from build123d import *

# Parameters (mm, degrees)
SKETCH1_W                                = 70.104
SKETCH1_H                                = 38.1
RECTANGULAR_BASE_DEPTH                   = 3.175
SKETCH2_R                                = 34.29
CIRCULAR_BASE_ADD_ON_DEPTH               = 3.175
HOLE_FOR_SERVO_ARM_DEPTH                 = 4.175
TAB_DEPTH                                = 3.175
CIRCULAR_PATTERN_OF_SERVO_ARM_HOLE_COUNT = 4
SKETCH6_R                                = 11.43
CUT_EXTRUDE2_DEPTH                       = 4.175


with BuildPart() as part:
    # Sketch1 → rectangular base (new body)
    with BuildSketch(Plane(origin=(0, 0, 0), x_dir=(1, 0, 0), z_dir=(0, 1, 0))):
        Rectangle(SKETCH1_W, SKETCH1_H)
    extrude(amount=RECTANGULAR_BASE_DEPTH)

    # Sketch2 → circular base add on (add)
    with BuildSketch(Plane(origin=(0, 3.175, 0), x_dir=(1, 0, 0), z_dir=(0, 1, 0))):
        Circle(SKETCH2_R)
    extrude(amount=-CIRCULAR_BASE_ADD_ON_DEPTH)

    # Sketch3 → hole for servo arm (cut, through all)
    with BuildSketch(Plane(origin=(0, 3.175, 0), x_dir=(1, 0, 0), z_dir=(0, 1, 0))):
        with BuildLine():
            Line((-2.54, 18.306077), (-4.445, 5.588))
            Line((-4.445, 5.588), (-5.881840979, 4.151159021))
            Line((-5.881840979, 4.151159021), (0, 0))
            Line((0, 0), (5.881840979, 4.151159021))
            Line((5.881840979, 4.151159021), (4.445, 5.588))
            Line((4.445, 5.588), (2.54, 18.306077))
            ThreePointArc((2.54, 18.306077), (0, 20.366046175), (-2.54, 18.306077))
        make_face()
    hole_for_servo_arm = extrude(amount=-HOLE_FOR_SERVO_ARM_DEPTH, mode=Mode.SUBTRACT)

    # Sketch4 → tab (add)
    with BuildSketch(Plane(origin=(0, 3.175, 0), x_dir=(1, 0, 0), z_dir=(0, 1, 0))):
        Polygon((-35.052, 0), (-35.052, 3.175), (-38.2778, 3.175), (-38.2778, -3.175), (-35.052, -3.175), align=None)
    tab = extrude(amount=-TAB_DEPTH)

    # Mirror1: tab across plane
    add(tab.mirror(Plane(origin=(0, 0, 0), x_dir=(0, 0, 1), z_dir=(1, 0, 0))))

    # Circular pattern of servo arm hole: hole for servo arm ×4 about axis
    circular_pattern_of_servo_arm_hole_axis = Axis((0, 0, 0), (0, 1, 0))
    for i in range(1, CIRCULAR_PATTERN_OF_SERVO_ARM_HOLE_COUNT):
        add(hole_for_servo_arm.rotate(circular_pattern_of_servo_arm_hole_axis, i * 360 / CIRCULAR_PATTERN_OF_SERVO_ARM_HOLE_COUNT), mode=Mode.SUBTRACT)

    # Sketch6 → Cut-Extrude2 (cut, through all)
    with BuildSketch(Plane(origin=(0, 3.175, 0), x_dir=(1, 0, 0), z_dir=(0, 1, 0))):
        Circle(SKETCH6_R)
    extrude(amount=-CUT_EXTRUDE2_DEPTH, mode=Mode.SUBTRACT)


solid = part.part
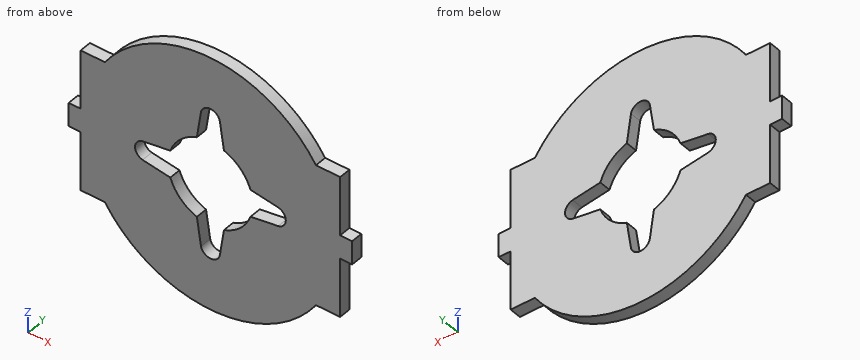
Geometry check sheet. Reference: the model listing, model coordinates, mm. Round coordinates to 2 decimals unless told otherwise and drop trailing zeros. Order: outer loops, then holes, each group sorted by start corner. A loop starts at its lowest first (then second) coordinate and runs counter-clockwise, first axis right, second up. Notation, with made-up numbers: M -33.5,18 L 2.5,18 A32 cw 2.5,53 Z; hole C 6.25,3.25 d2. An arc over 180 degrees is marked long. Answer in a Markdown table with one row per item. Add a question column.
Item 1: Sectioned sample at C-C, the plane x = -29.5. Enter the section's corners in (y, z) (3 decimals).
Item 2: Material ranges on L1, parallel to X at y = 1.8, z = 0; L2, parallel to X at y = 0.1, z = -0.5; L3, parallel to Z at x = 16, y = 1.65, recorded low to high. Write a range as [from, to].
Item 3: Sectioned sample at B-B, the plane z = -15. Enter the section's corners in (x, y) (3 decimals), plus the area to 3 significant figures.
Item 4: Depth check by flat-ended pin: pin 1 Ø1 at (y, z) = (1.5, -9.5) entering from -X; pin 2 Ø1.5 at (x, y) = (3.5, 1) entering from -Z; pin 3 Ø1 at (x, y) = (-12.5, 1) entering from -Z; pin 4 Ø8 at (x, z) = (-26, -25) entering from -Y. Enter the tip coordinate at first touch or a pass-through.
Item 5: Sectioned sample at D-D, the plane z = 14. Enter the section's corners in (x, y) (3 decimals).
Filled in:
| question | item | result |
|---|---|---|
| 1 | outline | M 0,-19.05 L 3.175,-19.05 L 3.175,19.05 L 0,19.05 Z |
| 2 | L1 | x = [-38.28, -20.37], [20.37, 38.28] |
| 2 | L2 | x = [-38.28, -20.32], [20.32, 38.28] |
| 2 | L3 | z = [-30.33, -2.89], [2.89, 30.33] |
| 3 | outline | M -35.052,0 L -3.035,0 L -3.035,3.175 L -35.052,3.175 Z; M 3.035,0 L 35.052,0 L 35.052,3.175 L 3.035,3.175 Z |
| 3 | area | 203 mm² |
| 4 | pin 1 | stops at x = -35.05 |
| 4 | pin 2 | stops at z = -34.18 |
| 4 | pin 3 | stops at z = -32.12 |
| 4 | pin 4 | stops at y = 0 |
| 5 | outline | M -35.052,0 L -3.185,0 L -3.185,3.175 L -35.052,3.175 Z; M 3.185,0 L 35.052,0 L 35.052,3.175 L 3.185,3.175 Z |
